Check sheet for the modelled part. Datum: model origin and axes. Units: mm. Coordinates: 2 decimals unless noted, no trailing zeros. Write each loop counter-clockwise with the first axis right and the second up, starting at its lowest first coordinate (ties: lowest second). Pieces come first, ordered by that corner, then holes. Notation, with made-up numbers: M 15.5,89 L 20.5,89 A11 cw 20.5,98 Z; hole C 11.5,69 d7. An arc over 180 degrees is marked long. Answer as CSV lines item,"result". Start each with the question number.
Q1. Thickness scan on line 1 along X through (y, z) = (-45.5, 3.1); line 2 along X through (y, z) = (15, 2); line 3 along X through (y, z) = (-14.5, 1.1). Record the ranges inside material, lowest first. Write a range as from..to.
Q2. Sectioned sample at B-B, the plane x = 95.5. Record the cut outline in (y, z).
Q3. Sectioned sample at A-A, the plane x = -116. Record the cut outline in (y, z), then the cut area to 3 significant figures.
Q4. Sectioned sample at C-C, the plane z = 1.8. Count the separate pieces of the cut face and the enclosed holes in it, then the cut area to 3 significant figures.
Q5. Depth check by flat-ended pin: pin 1 Ø2 at (y, z) = (88.5, 3) entering from +X; pin 2 Ø1.5 at (x, z) = (-56.5, 4) entering from -Y; pin 3 Ø6 at (x, y) = (-70.5, 16) entering from -Z; pin 4 Ø2 at (x, z) = (58, 1.5) entering from +Y. Enter the tip coordinate at first touch or a pass-through.
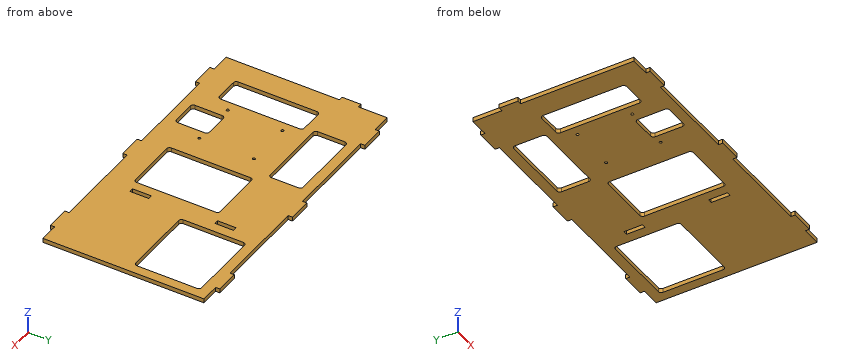
Autodesk Fusion 360 part; units mm, degrees
sketch "Sketch1" plane through (0, 0, 0) normal (0, 0, 1) x (1, 0, 0)
  line L0 (160, -90) -> (-160, -90)
  line L1 (-160, -90) -> (-160, 90)
  line L2 (-160, 90) -> (160, 90)
  line L3 (160, 90) -> (160, -90)
  line L4 (160, -90) -> (-160, 90) construction
  line L5 (-160, -90) -> (160, 90) construction
  line L6 (170, 85.5) -> (-180, 85.5) construction
  line L7 (-180, -85.5) -> (170, -85.5) construction
  line L8 (-155.5, 90) -> (-155.5, -90)
  line L9 (-160, 90) -> (-135, 90)
  line L10 (-135, 90) -> (-135, 85.5)
  line L11 (-135, 85.5) -> (-160, 85.5)
  line L12 (-160, 85.5) -> (-160, 90)
  line L13 (-160, -90) -> (-135, -90)
  line L14 (-135, -90) -> (-135, -85.5)
  line L15 (-135, -85.5) -> (-160, -85.5)
  line L16 (-160, -85.5) -> (-160, -90)
  line L17 (-110, -90) -> (-10, -90)
  line L18 (-10, -90) -> (-10, -85.5)
  line L19 (-10, -85.5) -> (-110, -85.5)
  line L20 (-110, -85.5) -> (-110, -90)
  line L21 (-10, -90) -> (15, -90)
  line L22 (15, -90) -> (15, -85.5)
  line L23 (15, -85.5) -> (-10, -85.5)
  line L24 (-10, -85.5) -> (-10, -90)
  line L25 (15, -90) -> (115, -90)
  line L26 (115, -90) -> (115, -85.5)
  line L27 (115, -85.5) -> (15, -85.5)
  line L28 (15, -85.5) -> (15, -90)
  line L29 (115, -90) -> (140, -90)
  line L30 (140, -90) -> (140, -85.5)
  line L31 (140, -85.5) -> (115, -85.5)
  line L32 (115, -85.5) -> (115, -90)
  line L33 (-135, 85.5) -> (-110, 85.5)
  line L34 (-110, 85.5) -> (-110, 90)
  line L35 (-110, 90) -> (-135, 90)
  line L36 (-135, 90) -> (-135, 85.5)
  line L37 (-110, 85.5) -> (-10, 85.5)
  line L38 (-10, 85.5) -> (-10, 90)
  line L39 (-10, 90) -> (-110, 90)
  line L40 (-110, 90) -> (-110, 85.5)
  line L41 (-10, 85.5) -> (15, 85.5)
  line L42 (15, 85.5) -> (15, 90)
  line L43 (15, 90) -> (-10, 90)
  line L44 (-10, 90) -> (-10, 85.5)
  line L45 (15, 85.5) -> (115, 85.5)
  line L46 (115, 85.5) -> (115, 90)
  line L47 (115, 90) -> (15, 90)
  line L48 (15, 90) -> (15, 85.5)
  line L49 (115, 85.5) -> (140, 85.5)
  line L50 (140, 85.5) -> (140, 90)
  line L51 (140, 90) -> (115, 90)
  line L52 (115, 90) -> (115, 85.5)
  line L53 (140, 85.5) -> (160, 85.5)
  line L54 (160, 85.5) -> (160, 90)
  line L55 (160, 90) -> (140, 90)
  line L56 (140, 90) -> (140, 85.5)
  line L57 (140, -90) -> (160, -90)
  line L58 (160, -90) -> (160, -85.5)
  line L59 (160, -85.5) -> (140, -85.5)
  line L60 (140, -85.5) -> (140, -90)
  line L61 (-160, 55) -> (-155.5, 55)
  line L62 (-155.5, 55) -> (-155.5, 35)
  line L63 (-155.5, 35) -> (-160, 35)
  line L64 (-160, 35) -> (-160, 55)
  line L65 (-160, -35) -> (-155.5, -35)
  line L66 (-155.5, -35) -> (-155.5, -55)
  line L67 (-155.5, -55) -> (-160, -55)
  line L68 (-160, -55) -> (-160, -35)
  line L69 (55, 100) -> (55, -100) construction
  line L70 (59.5, 100) -> (59.5, -100) construction
  line L71 (55, 55) -> (59.5, 55)
  line L72 (59.5, 55) -> (59.5, 35)
  line L73 (59.5, 35) -> (55, 35)
  line L74 (55, 35) -> (55, 55)
  line L75 (55, -35) -> (59.5, -35)
  line L76 (59.5, -35) -> (59.5, -55)
  line L77 (59.5, -55) -> (55, -55)
  line L78 (55, -55) -> (55, -35)
  line L79 (-40.5, -43) -> (-89.5, -43) construction
  line L80 (-89.5, -43) -> (-89.5, 15) construction
  line L81 (-89.5, 15) -> (-40.5, 15) construction
  line L82 (-40.5, 15) -> (-40.5, -43) construction
  line L83 (-40.5, -43) -> (-89.5, 15) construction
  line L84 (-89.5, -43) -> (-40.5, 15) construction
  circle A0 centre (-40.5, 15) radius 1.4
  circle A1 centre (-89.5, 15) radius 1.4
  circle A2 centre (-89.5, -43) radius 1.4
  circle A3 centre (-40.5, -43) radius 1.4
  line L85 (-53, -75) -> (-77, -75)
  line L86 (-80, -72) -> (-80, -43)
  line L87 (-77, -40) -> (-53, -40)
  line L88 (-50, -43) -> (-50, -72)
  line L89 (-50, -75) -> (-80, -40) construction
  line L90 (-80, -75) -> (-50, -40) construction
  arc A4 (-77, -40) -> (-80, -43) centre (-77, -43) ccw
  arc A5 (-50, -43) -> (-53, -40) centre (-53, -43) ccw
  arc A6 (-80, -72) -> (-77, -75) centre (-77, -72) ccw
  arc A7 (-53, -75) -> (-50, -72) centre (-53, -72) ccw
  line L91 (-28, 40) -> (-102, 40)
  line L92 (-105, 43) -> (-105, 72)
  line L93 (-102, 75) -> (-28, 75)
  line L94 (-25, 72) -> (-25, 43)
  line L95 (-25, 40) -> (-105, 75) construction
  line L96 (-105, 40) -> (-25, 75) construction
  arc A8 (-102, 75) -> (-105, 72) centre (-102, 72) ccw
  arc A9 (-25, 72) -> (-28, 75) centre (-28, 72) ccw
  arc A10 (-105, 43) -> (-102, 40) centre (-102, 43) ccw
  arc A11 (-28, 40) -> (-25, 43) centre (-28, 43) ccw
  line L97 (147, 5) -> (73, 5)
  line L98 (70, 8) -> (70, 72)
  line L99 (73, 75) -> (147, 75)
  line L100 (150, 72) -> (150, 8)
  line L101 (150, 5) -> (70, 75) construction
  line L102 (70, 5) -> (150, 75) construction
  arc A12 (70, 8) -> (73, 5) centre (73, 8) ccw
  arc A13 (73, 75) -> (70, 72) centre (73, 72) ccw
  arc A14 (150, 72) -> (147, 75) centre (147, 72) ccw
  arc A15 (147, 5) -> (150, 8) centre (147, 8) ccw
  line L103 (42, -60) -> (-12, -60)
  line L104 (-15, -57) -> (-15, 27)
  line L105 (-12, 30) -> (42, 30)
  line L106 (45, 27) -> (45, -57)
  line L107 (45, -60) -> (-15, 30) construction
  line L108 (-15, -60) -> (45, 30) construction
  arc A16 (-12, 30) -> (-15, 27) centre (-12, 27) ccw
  arc A17 (45, 27) -> (42, 30) centre (42, 27) ccw
  arc A18 (-15, -57) -> (-12, -60) centre (-12, -57) ccw
  arc A19 (42, -60) -> (45, -57) centre (42, -57) ccw
  line L109 (-103, -60) -> (-127, -60)
  line L110 (-130, -57) -> (-130, 27)
  line L111 (-127, 30) -> (-103, 30)
  line L112 (-100, 27) -> (-100, -57)
  line L113 (-100, -60) -> (-130, 30) construction
  line L114 (-130, -60) -> (-100, 30) construction
  arc A20 (-127, 30) -> (-130, 27) centre (-127, 27) ccw
  arc A21 (-100, 27) -> (-103, 30) centre (-103, 27) ccw
  arc A22 (-130, -57) -> (-127, -60) centre (-127, -57) ccw
  arc A23 (-103, -60) -> (-100, -57) centre (-103, -57) ccw
  point P0 (-65, -14)
  point P1 (-65, -57.5)
  point P2 (-65, 57.5)
  point P3 (110, 40)
  point P4 (15, -15)
  point P5 (-115, -15)
  dimension "d1" = 320
  dimension "d2" = 180
  dimension "d3" = 4.5
  dimension "d4" = 4.5
  dimension "d5" = 4.5
  dimension "d6" = 25
  dimension "d7" = 25
  dimension "d8" = 100
  dimension "d9" = 25
  dimension "d10" = 25
  dimension "d11" = 100
  dimension "d12" = 25
  dimension "d13" = 25
  dimension "d14" = 100
  dimension "d15" = 25
  dimension "d16" = 100
  dimension "d17" = 25
  dimension "d18" = 20
  dimension "d19" = 20
  dimension "d20" = 35
  dimension "d21" = 35
  dimension "d22" = 215
  dimension "d23" = 4.5
  dimension "d24" = 20
  dimension "d25" = 20
  dimension "d26" = 35
  dimension "d27" = 35
  dimension "d28" = 49
  dimension "d29" = 58
  dimension "d30" = 76
  dimension "d31" = 120
  dimension "d32" = 2.8
  dimension "d33" = 2.8
  dimension "d34" = 2.8
  dimension "d35" = 2.8
  dimension "d46" = 30
  dimension "d47" = 35
  dimension "d48" = 3
  dimension "d49" = 3
  dimension "d50" = 3
  dimension "d51" = 3
  dimension "d52" = 80
  dimension "d53" = 35
  dimension "d54" = 25
  dimension "d55" = 3
  dimension "d56" = 3
  dimension "d57" = 3
  dimension "d58" = 3
  dimension "d65" = 80
  dimension "d66" = 70
  dimension "d67" = 3
  dimension "d68" = 3
  dimension "d69" = 3
  dimension "d70" = 3
  dimension "d71" = 3
  dimension "d72" = 3
  dimension "d73" = 3
  dimension "d74" = 3
  dimension "d75" = 3
  dimension "d76" = 3
  dimension "d77" = 3
  dimension "d78" = 3
  dimension "d103" = 10.5
  dimension "d104" = 10.5
  dimension "d105" = 10.5
extrude "Extrude1" add sketch "Sketch1" along normal blind 4.5 contours L0 L26 L29 L30 L31 L32 L60 | L0 L3 L8 L11 L14 L15 L19 L20 L23 L27 L31 L33 L37 L41 L45 L49 L53 L59 L62 L66 | L0 L18 L21 L22 L23 L24 L28 | L2 L46 L49 L50 L51 L52 L56 | L2 L38 L41 L42 L43 L44 L48 | L2 L10 L33 L34 L35 L36 L40 | L1 L8 L61 L62 L63 L64
move_face "OffsetFaces1" offset -0.1 6 faces at (140, -88.5, 1.5) (15, -88.5, 1.5) (-110, -87, 1.5) (140, 87, 1.5) (15, 87, 1.5) (-110, 87, 1.5)
move_face "OffsetFaces2" offset -0.1 6 faces at (115, -88.5, 1.5) (-10, -88.5, 1.5) (-135, -88.5, 1.5) (-135, 88.5, 1.5) (-10, 87, 1.5) (115, 87, 1.5)
move_face "OffsetFaces5" offset -0.1 1 faces at (-157, 35, 1.5)
move_face "OffsetFaces6" offset -0.1 1 faces at (-158.5, 55, 1.5)
Output:
1,line 1,"x = -155.5..-130, -100..-80, -50..-15, 45..55, 59.5..160"
1,line 2,"x = -155.5..-130, -100..-90.9, -88.1..-41.9, -39.1..-15, 45..70, 150..160"
1,line 3,"x = -155.5..-130, -100..-15, 45..160"
2,outline,"M -85.5,0 L 5,0 L 5,4.5 L -85.5,4.5 Z; M 75,0 L 85.5,0 L 85.5,4.5 L 75,4.5 Z"
3,outline,"M -90,0 L -60,0 L -60,4.5 L -90,4.5 Z; M 30,0 L 90,0 L 90,4.5 L 30,4.5 Z"
3,area,"405 mm^2"
4,separate pieces,"1"
4,enclosed holes,"11"
4,area,"37,000 mm^2"
5,pin 1,"stops at x = 139.9"
5,pin 2,"stops at y = -85.5"
5,pin 3,"stops at z = 0"
5,pin 4,"stops at y = 85.5"
